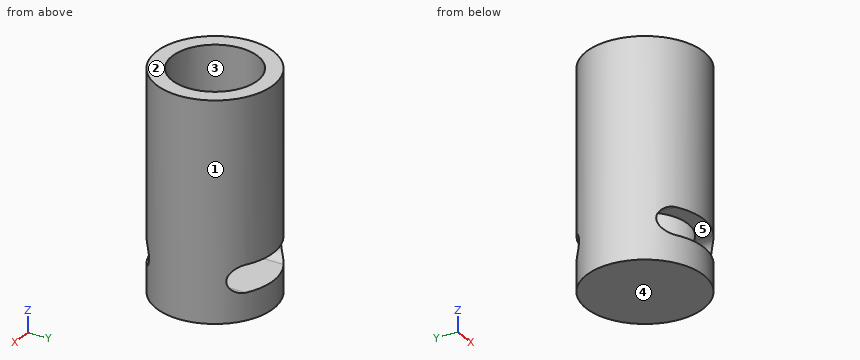
```python
from build123d import *

# Parameters (mm, degrees)
F0_R     = 6.5
F1_DEPTH = 4
F2_R     = 6.5
F2_R_2   = 4.75
F3_DEPTH = 20
F6_DEPTH = 25


with BuildPart() as f1:
    # F0 (on Top) → F1 (new body)
    with BuildSketch(Plane.XY):
        Circle(F0_R)
    extrude(amount=F1_DEPTH)

    # F2 (on face) → F3 (join)
    with BuildSketch(Plane.XY.offset(4)):
        Circle(F2_R)
        Circle(F2_R_2, mode=Mode.SUBTRACT)
    extrude(amount=F3_DEPTH)

    # F5 (on offset) → F6 (cut)
    with BuildSketch(Plane.XZ.offset(10)):
        with BuildLine():
            ThreePointArc((-1.85, 4.5), (-2.2893398282, 5.5606601718), (-3.35, 6))
            Line((-3.35, 6), (-3.35, 3))
            ThreePointArc((-3.35, 3), (-2.2893398282, 3.4393398282), (-1.85, 4.5))
        make_face()
        with BuildLine():
            Line((3.35, 6), (-3.35, 6))
            ThreePointArc((-3.35, 6), (-2.2893398282, 5.5606601718), (-1.85, 4.5))
            ThreePointArc((-1.85, 4.5), (-2.2893398282, 3.4393398282), (-3.35, 3))
            Line((-3.35, 3), (3.35, 3))
            ThreePointArc((3.35, 3), (1.85, 4.5), (3.35, 6))
        make_face()
        with BuildLine():
            Line((-3.35, 3), (-3.35, 6))
            ThreePointArc((-3.35, 6), (-4.85, 4.5), (-3.35, 3))
        make_face()
        with BuildLine():
            ThreePointArc((4.85, 4.5), (4.4106601718, 5.5606601718), (3.35, 6))
            Line((3.35, 6), (3.35, 3))
            ThreePointArc((3.35, 3), (4.4106601718, 3.4393398282), (4.85, 4.5))
        make_face()
        with BuildLine():
            Line((3.35, 3), (3.35, 6))
            ThreePointArc((3.35, 6), (1.85, 4.5), (3.35, 3))
        make_face()
    extrude(amount=-F6_DEPTH, mode=Mode.SUBTRACT)


solid = f1.part
```
Build history of the part. All positions in model axes, mm. Face numbers are marked on the shaded views. A direction names the side the tool comes from. Give positions to 0.01 mm unless a question says otherwise; leave off trailing zeros. Loops run counter-clockwise (first coordinate to the right, second up) from the corner with the lowest first, then second, coordinate; pieces in that order, holes last.
1) Two-plate mould, pull along Y, no slides. Class the marked faces 1, 2 and 3: released by +Y, released by -Y, zero draft, split by the parting line, or undercut.
Values follow:
face 1: split by the parting line
face 2: zero draft
face 3: undercut
2) Drop flat-ended pins along their axis: P1, Ø1.5, axis at y = 3, z = 3.5, coming from the -X side; P2, Ø5, axis at x = 2.5, y = -3.5, coming from the +Z side; P3, Ø1, axis at x = 3, y = -2, coming from the +Z side; P4, Ø1.5, axis at x = 3, z = 20, coming from the +Y side. Give the stop position or say it passes through.
Values follow:
P1: stops at x = -6.1
P2: stops at z = 24
P3: stops at z = 3.01
P4: stops at y = 6.1
3) Band-saw the part on A-A on x = 0. List the corners of the cut face in (y, z), then the cut area to 3 significant figures.
Values follow:
outline: (-6.5, 0) - (6.5, 0) - (6.5, 3) - (-6.5, 3) - close; (-6.5, 6) - (-4.75, 6) - (-4.75, 24) - (-6.5, 24) - close; (4.75, 6) - (6.5, 6) - (6.5, 24) - (4.75, 24) - close
area: 102 mm2
4) Band-saw the part on B-B on y = 0. List the corners of the cut face in (x, z), then the cut area to 3 significant figures.
Values follow:
outline: (-6.5, 0) - (6.5, 0) - (6.5, 24) - (4.75, 24) - (4.75, 5.04) arc R1.5 cw to (3.35, 3) - (-3.35, 3) arc R1.5 cw to (-4.75, 5.04) - (-4.75, 24) - (-6.5, 24) - close
area: 113 mm2
5) Band-saw the part on D-D on x = -2. List the corners of the cut face in (y, z), then the cut area to 3 significant figures.
Values follow:
outline: (-6.18, 0) - (6.18, 0) - (6.18, 3) - (-6.18, 3) - close; (-6.18, 6) - (-4.31, 6) - (-4.31, 24) - (-6.18, 24) - close; (4.31, 6) - (6.18, 6) - (6.18, 24) - (4.31, 24) - close
area: 105 mm2
6) Band-saw the part on C-C on z = 16.25. List the corners of the cut face in (x, y), then the cut area to 4 significant figures.
Values follow:
outline: circle Ø13 at (0, 0); hole circle Ø9.5 at (0, 0)
area: 61.85 mm2
7) Probe line 1 along Y through (x, z) = (0, 9.75); line 2 along Z through (x, y) = (-2, -4.5); line 3 along Y through (x, z) = (-2, 19.5). List the from-to ranges inside material, lowest first.
Values follow:
line 1: y = -6.5 to -4.75, 4.75 to 6.5
line 2: z = 0 to 3, 6 to 24
line 3: y = -6.18 to -4.31, 4.31 to 6.18
8) 3-axis set-ups, long thin cutter, end or side, ignore diameter. For the marked faces 4 and 5: which of +Z, -Z, +X, -X, +Y, -Y reach the whole face in a straight line?
Values follow:
face 4: -Z, +X, -X, +Y, -Y
face 5: +Y, -Y
